Job drawing, mm, ordinate dimensions from the low corner. One solid piece. Give positions to 0.01 mm unless a question says otherwise; leave off trailing zeros. Write each loop counter-clockwise with the first axis right and the second up, starting at its lowest first coordinate (ties: lowest second). Pieces come first, ordered by that corner, then holes. Notation, with made-up numbers: (47.25, 39.25) - (84.25, 39.25) arc R29 ccw to (84.25, 72.25) - close; hole circle Ø6 at (60.25, 66). An arc over 180 degrees is marked (long way). Put each result on its own line as item: value. Start each with the question number.
1. Cut at C-C on x = 34. List the corners of the cut face in (y, z).
2. Wall check: line 1 (X direction, y = 23.5, z = 1.9) (1 decimal); line 2 (X direction, y = 53, z = 0.85) (1 decimal); line 3 (Y direction, x = 29, z = 3.35) (1 decimal). Give the ranges that are in metal, low to high.
3. Cut at A-A on z = 2.9. List the corners of the cut face in (x, y) (1 decimal), and give its area (3 significant figures).
4. Drop flat-ended pins along their axis: pin 1 (2 mm diameter, centred on y = 50.5, z = 4, fed in from +X); pin 2 (2 mm diameter, centred on y = 85.5, z = 2.5, fed in from -X) (1 decimal); pin 3 (2 mm diameter, centred on y = 75.5, z = 1, fed in from +X) (1 decimal); pin 4 (3 mm diameter, centred on x = 39, y = 101.5, fed in from -Z). Give the stop position or say it passes through.
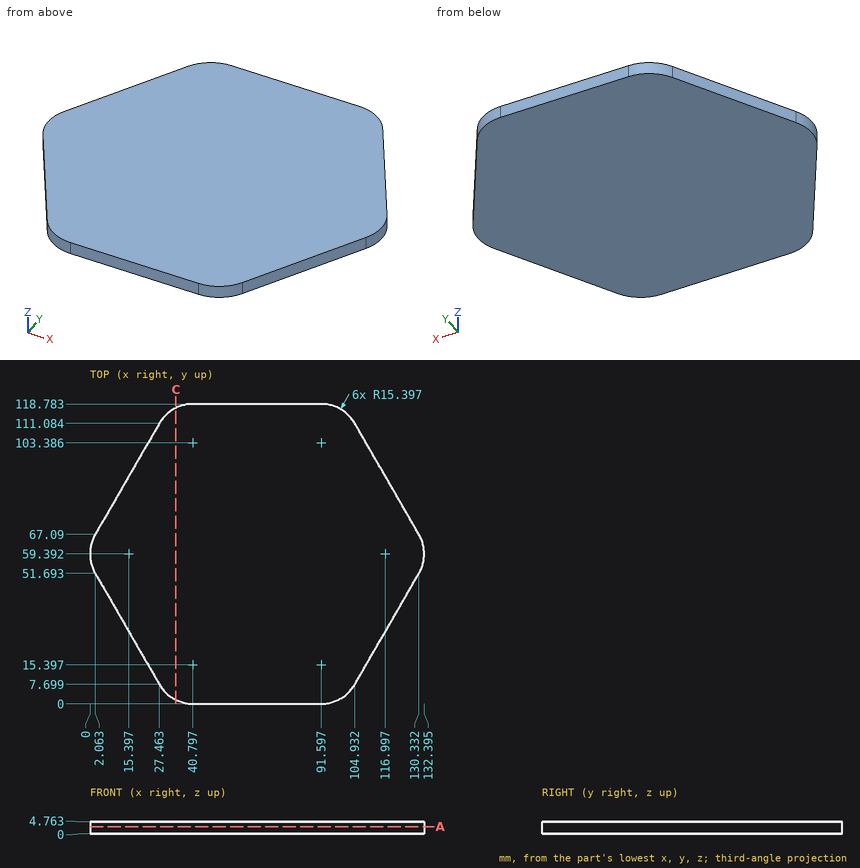
Report:
1. outline: (1.58, 0) - (117.2, 0) - (117.2, 4.76) - (1.58, 4.76) - close
2. line 1: x = 18.3 to 114.1
2. line 2: x = 1.4 to 131
2. line 3: y = 5.5 to 113.3
3. outline: (2.1, 51.7) - (27.5, 7.7) arc R15.4 ccw to (40.8, 0) - (91.6, 0) arc R15.4 ccw to (104.9, 7.7) - (130.3, 51.7) arc R15.4 ccw to (130.3, 67.1) - (104.9, 111.1) arc R15.4 ccw to (91.6, 118.8) - (40.8, 118.8) arc R15.4 ccw to (27.5, 111.1) - (2.1, 67.1) arc R15.4 ccw to start
3. area: 12,100 mm²
4. pin 1: stops at x = 130.22
4. pin 2: stops at x = 12.1
4. pin 3: stops at x = 126.1
4. pin 4: stops at z = 0
